Input: part model. Units: mm. Frame: model coordinates. A direction names the side the tool comes from. Round coordinates to 2 decimals unless told otherwise and drop trailing zeros. Loops run counter-clockwise (first coordinate to the right, second up) from the corner with the lowest first, then second, coordinate; pieces in that order, holes last. Notation, with made-up numbers: (75.5, 80.25) - (134.5, 80.25) arc R36 cw to (134.5, 119.25) - close; hole circle Ø4 at (-29, 60). An arc over 180 degrees is marked (long way). Write each question's results on one line, items separated by ' | '.
from build123d import *

# Parameters (mm, degrees)
BOSS_EXTRUDE1_DEPTH = 14
CUT_EXTRUDE1_REACH  = 8
SKETCH2_R           = 2.5
SKETCH3_R           = 1.5
CUT_EXTRUDE2_DEPTH  = 31


with BuildPart() as part:
    # Sketch1 → Boss-Extrude1 (new body)
    with BuildSketch(Plane.XY):
        with BuildLine():
            Line((-0.95630186, 29.8), (-0.95630186, 21.397213521))
            ThreePointArc((-0.95630186, 21.397213521), (0, 12.5), (0.95630186, 21.397213521))
            Line((0.95630186, 21.397213521), (0.95630186, 29.8))
            Line((0.95630186, 29.8), (9, 29.8))
            Line((9, 29.8), (9, 3))
            Line((9, 3), (21, 3))
            Line((21, 3), (21, -3))
            Line((21, -3), (-21, -3))
            Line((-21, -3), (-21, 3))
            Line((-21, 3), (-9, 3))
            Line((-9, 3), (-9, 29.8))
            Line((-9, 29.8), (-0.95630186, 29.8))
        make_face()
    extrude(amount=BOSS_EXTRUDE1_DEPTH)

    # Sketch2 → Cut-Extrude1 (cut, up to next)
    with BuildSketch(Plane(origin=(0, 3, 0), x_dir=(1, 0, 0), z_dir=(0, 1, 0)), mode=Mode.PRIVATE) as cut_extrude1_sk1:
        with Locations((-16, -7)):
            Circle(SKETCH2_R)
    cut_extrude1_tool1 = extrude(cut_extrude1_sk1.sketch, amount=-CUT_EXTRUDE1_REACH, mode=Mode.PRIVATE) & part.part
    add(cut_extrude1_tool1.solids().sort_by_distance((-16, 3, 7))[0], mode=Mode.SUBTRACT)
    # Sketch2 → Cut-Extrude1 (cut, up to next)
    with BuildSketch(Plane(origin=(0, 3, 0), x_dir=(1, 0, 0), z_dir=(0, 1, 0)), mode=Mode.PRIVATE) as cut_extrude1_sk2:
        with Locations((16, -7)):
            Circle(SKETCH2_R)
    cut_extrude1_tool2 = extrude(cut_extrude1_sk2.sketch, amount=-CUT_EXTRUDE1_REACH, mode=Mode.PRIVATE) & part.part
    add(cut_extrude1_tool2.solids().sort_by_distance((16, 3, 7))[0], mode=Mode.SUBTRACT)

    # Sketch3 → Cut-Extrude2 (cut, through all)
    with BuildSketch(Plane.ZY.offset(9)):
        with Locations((7, 25.3)):
            Circle(SKETCH3_R)
    extrude(amount=-CUT_EXTRUDE2_DEPTH, mode=Mode.SUBTRACT)


solid = part.part
1. Contact query for flat-ended pins moving along their axis: pin 1 (4 mm diameter, centred on y = 13.5, z = 5, fed in from -X); pin 2 (7 mm diameter, centred on y = 15, z = 5.5, fed in from +X); pin 3 (3.5 mm diameter, centred on x = -17, z = 4.5, fed in from +Y). Output: stop coordinate, or through.
Answer:
pin 1: x = -9 | pin 2: x = 9 | pin 3: y = 3
2. Mould query, pull axis Z, two halves, no side actions, for faces 1 (the flat face through (5, 29.8, 7)), 2 (the cylindrical face through (-18.5, 0, 6.9)), 3 (the flat face through (0, 6, 0)), 4 (the cylindrical face through (13.5, 0, 6.9)). Classes: pulls with the +Z half, pulls with the -Z half, needs draft (parallel to the pull), parting line crosses it, or undercut.
Answer:
face 1: needs draft | face 2: undercut | face 3: pulls with the -Z half | face 4: undercut
3. Section query B-B, the plane x = -16. Output: boundary loops of the cut face in (y, z).
Answer:
outline: (-3, 0) - (3, 0) - (3, 4.5) - (-3, 4.5) - close; (-3, 9.5) - (3, 9.5) - (3, 14) - (-3, 14) - close
4. Section query C-C, the plane y = 17. Output: boundary loops of the cut face in (x, z).
Answer:
outline: (-9, 0) - (-4.5, 0) - (-4.5, 14) - (-9, 14) - close; (4.5, 0) - (9, 0) - (9, 14) - (4.5, 14) - close
5. Section query A-A, the plane z = 7. Output: boundary loops of the cut face in (x, y), plus the area to 3 significant figures.
Answer:
outline: (-21, -3) - (-18.5, -3) - (-18.5, 3) - (-21, 3) - close; (-13.5, -3) - (13.5, -3) - (13.5, 3) - (9, 3) - (9, 23.8) - (0.96, 23.8) - (0.96, 21.4) arc R4.5 cw (long way) to (-0.96, 21.4) - (-0.96, 23.8) - (-9, 23.8) - (-9, 3) - (-13.5, 3) - close; (-9, 26.8) - (-0.96, 26.8) - (-0.96, 29.8) - (-9, 29.8) - close; (0.96, 26.8) - (9, 26.8) - (9, 29.8) - (0.96, 29.8) - close; (18.5, -3) - (21, -3) - (21, 3) - (18.5, 3) - close | area: 547 mm^2
6. Line query: line 1 (X direction, y = -0.55, z = 7); line 2 (Z direction, x = 16, y = -1.45); line 3 (X direction, y = 27, z = 2.25). Output: solid intervals per line, ascending. Write a range as [from, to].
Answer:
line 1: [-21, -18.5], [-13.5, 13.5], [18.5, 21] | line 2: [0, 4.5], [9.5, 14] | line 3: [-9, -0.96], [0.96, 9]
7. Section query D-D, the plane y = 25.3. Output: boundary loops of the cut face in (x, z).
Answer:
outline: (-9, 0) - (-0.96, 0) - (-0.96, 5.5) - (-9, 5.5) - close; (-9, 8.5) - (-0.96, 8.5) - (-0.96, 14) - (-9, 14) - close; (0.96, 0) - (9, 0) - (9, 5.5) - (0.96, 5.5) - close; (0.96, 8.5) - (9, 8.5) - (9, 14) - (0.96, 14) - close
8. Set-up query: faces 5 (the flat face through (-0.956, 26, 5)), 6 (the cylindrical face through (-5.034, 23.836, 6.675)), 7 (the flat face through (-9, 16, 7)), 8 (the flat face through (9, 17, 7)). Return all of +Z, -Z, +X, -X, +Y, -Y with unobstructed straight access to the full face (end or side cutting, diameter ignored); none if empty.
Answer:
face 5: +Z, -Z, +Y | face 6: +X, -X | face 7: +Z, -Z, -X, +Y | face 8: +Z, -Z, +X, +Y
